The figure shows three views and two pictorial views of one solid part (mm, origin at its lowest corner). Answer the questions. Coordinates: 2 decimals unless noted, no trailing zeros. Write each loop counter-clockwise with the first axis right and the second up, starting at its lowest first coordinate (ties: lowest second). Pieces come first, ordered by that corner, then holes.
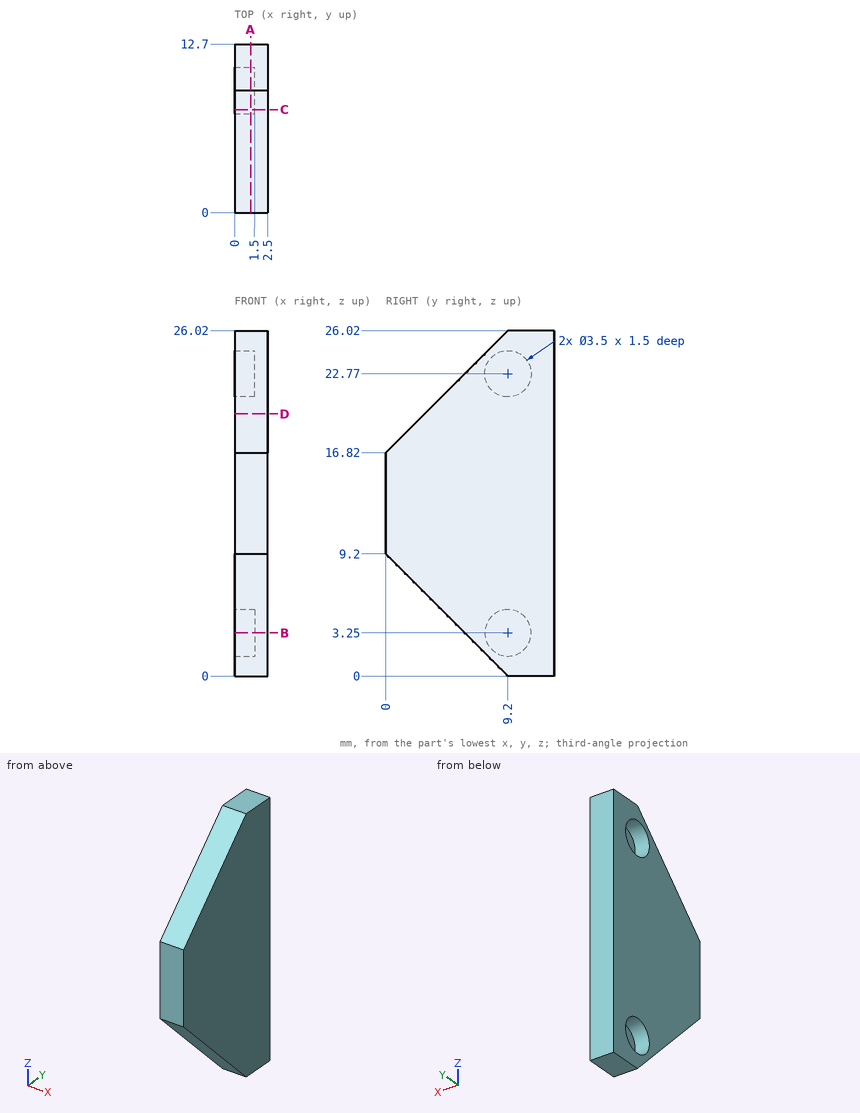
1. A flat-ended cylindrical pin translates along its axis: P1, Ø1, axis at y = 10, z = 2.5, coming from the -X side. Find the tip coordinate at first contact, or state that the pin passes through.
Results found:
P1: stops at x = 1.5
2. Find the intervals of material crossed by L1, parallel to Z at x = 0.8, y = 8; L2, parallel to Z at x = 0.8, y = 10; L3, parallel to Y at x = 0.4, z = 3.25, in increasing order.
Results found:
L1: z = 1.2 to 1.98, 4.52 to 21.5, 24.04 to 24.82
L2: z = 0 to 1.69, 4.81 to 21.21, 24.33 to 26.02
L3: y = 5.95 to 7.45, 10.95 to 12.7
3. Section D-D on z = 19.75 is taken. Give the vertices of the cut face in (x, y).
Results found:
outline: (0, 2.93) - (2.5, 2.93) - (2.5, 12.7) - (0, 12.7) - close
4. Section B-B on z = 3.25 is taken. Give the vertices of the cut face in (x, y).
Results found:
outline: (0, 5.95) - (2.5, 5.95) - (2.5, 12.7) - (0, 12.7) - (0, 10.95) - (1.5, 10.95) - (1.5, 7.45) - (0, 7.45) - close
5. Section A-A on x = 1.2 is taken. Give the vertices of the cut face in (y, z), then the cut area to 3 significant figures.
Results found:
outline: (0, 9.2) - (9.2, 0) - (12.7, 0) - (12.7, 26.02) - (9.2, 26.02) - (0, 16.82) - close; hole circle Ø3.5 at (9.2, 3.25); hole circle Ø3.5 at (9.2, 22.77)
area: 227 mm2
6. Section C-C on y = 7.75 is taken. Give the vertices of the cut face in (x, z), then the cut area to 3 significant figures.
Results found:
outline: (0, 1.45) - (2.5, 1.45) - (2.5, 24.57) - (0, 24.57) - (0, 23.75) - (1.5, 23.75) - (1.5, 21.79) - (0, 21.79) - (0, 4.23) - (1.5, 4.23) - (1.5, 2.27) - (0, 2.27) - close
area: 51.9 mm2
